Here's how the part is built. I have some questions about the finished solid (model axes, mm). A direction names the side the tool comes from. Coordinates: 2 decimals unless noted, no trailing zeros. Write each loop counter-clockwise with the first axis right and the second up, starting at its lowest first coordinate (ties: lowest second). Pieces come first, ordered by that corner, then holes.
(1) Thinking about a two-plate mould opening in X: for faces 1 (the flat face through (-2, -6, 1)), 2 (the cylindrical face through (-0.108, 5.812, 0.739)), 3 (the flat face through (5, -2, 1)), which applies, released by +X, released by -X, zero draft, split by the parting line, or undercut?
(2) Imagine slicing it at A-A, the plane x = -6.3. List the corners of the cut face in (y, z) for me, plus the area to 3 significant figures.
(3) Imagine slicing it at C-C, the plane z = -0.95. List the corners of the cut face in (x, y) for me, plus the area to 3 significant figures.
(4) Please list where these lines run through material, in increasing order: probe 1 along Y at (x, z) = (6.3, 0.5); probe 2 along Z at (x, y) = (9.25, 1.25); probe 3 along X at (y, z) = (0, -0.65).
(5) For pin 1 Ø2 at (x, z) = (-0.5, -1.5) entering from +Y; pin 2 Ø0.8 at (y, z) = (6, 1) entering from -X; pin 3 Ø3 at (x, y) = (0, -8) entering from -Z, each with a flat end and sliding along its axis, tell me the tip position at first contact or that it passes through.
(6) Imagine slicing it at D-D, the plane y = 0. State how many separate pieces and enclosed holes the cut face has, plus the area to 3 significant figures.
(7) Which directions (+Z, -Z, +X, -X, +Y, -Y) give clear straight access to the entire face, cutting with the end or side of a thin tool? Please do faces 4 (the flat face through (-6, -2, 1)), 5 (the flat face through (5, 2, 1)), 6 (the flat face through (2, -6, 1)), 7 (the flat face through (-6, 2, 1)).
```python
from build123d import *

# Parameters (mm, degrees)
COMPACT_HORN_CENTER_OD6P9_PROFILE_R        = 3.45
COMPACT_HORN_CENTER_OD6P9_DEPTH            = 1.5
HORIZONTAL_BLADES_ASSUMED_WIDTH4_PROFILE_W = 16.3
HORIZONTAL_BLADES_ASSUMED_WIDTH4_PROFILE_H = 4
HORIZONTAL_BLADES_ASSUMED_WIDTH4_DEPTH     = 1.5
VERTICAL_BLADES_ASSUMED_WIDTH4_PROFILE_W   = 4
VERTICAL_BLADES_ASSUMED_WIDTH4_PROFILE_H   = 16.3
VERTICAL_BLADES_ASSUMED_WIDTH4_DEPTH       = 1.5
ROUNDED_BLADE_TIPS_R                       = 2
ROUNDED_TIPS_SPAN20P3_DEPTH                = 1.5
HUB_PROJECTION2P5_TOTAL_HEIGHT4_START      = -2.5
HUB_PROJECTION2P5_TOTAL_HEIGHT4_PROFILE_R  = 3.45
HUB_PROJECTION2P5_TOTAL_HEIGHT4_DEPTH      = 2.5
PURCHASED_SPLINE_INTERNALS_OMITTED_START   = -50
PURCHASED_SPLINE_INTERNALS_OMITTED_PROFI_R = 2.55
PURCHASED_SPLINE_INTERNALS_OMITTED_DEPTH   = 65.570346598
UNMODIFIED_STOCK_PILOT_HOLES_START         = -50
UNMODIFIED_STOCK_PILOT_HOLES_PROFILE_R     = 0.5
UNMODIFIED_STOCK_PILOT_HOLES_DEPTH         = 65.570346598


with BuildPart() as part:
    # Compact_horn_center_OD6p9_profile → Compact_horn_center_OD6p9 (new body)
    with BuildSketch(Plane.XY):
        Circle(COMPACT_HORN_CENTER_OD6P9_PROFILE_R)
    extrude(amount=COMPACT_HORN_CENTER_OD6P9_DEPTH)

    # Horizontal_blades_assumed_width4_profile → Horizontal_blades_assumed_width4 (add)
    with BuildSketch(Plane.XY):
        Rectangle(HORIZONTAL_BLADES_ASSUMED_WIDTH4_PROFILE_W, HORIZONTAL_BLADES_ASSUMED_WIDTH4_PROFILE_H)
    extrude(amount=HORIZONTAL_BLADES_ASSUMED_WIDTH4_DEPTH)

    # Vertical_blades_assumed_width4_profile → Vertical_blades_assumed_width4 (add)
    with BuildSketch(Plane.XY):
        Rectangle(VERTICAL_BLADES_ASSUMED_WIDTH4_PROFILE_W, VERTICAL_BLADES_ASSUMED_WIDTH4_PROFILE_H)
    extrude(amount=VERTICAL_BLADES_ASSUMED_WIDTH4_DEPTH)

    # Rounded_blade_tips → Rounded_tips_span20p3 (add)
    with BuildSketch(Plane.XY):
        with Locations((8.15, 0)):
            Circle(ROUNDED_BLADE_TIPS_R)
        with Locations((-8.15, 0)):
            Circle(ROUNDED_BLADE_TIPS_R)
        with Locations((0, 8.15)):
            Circle(ROUNDED_BLADE_TIPS_R)
        with Locations((0, -8.15)):
            Circle(ROUNDED_BLADE_TIPS_R)
    extrude(amount=ROUNDED_TIPS_SPAN20P3_DEPTH)

    # Hub_projection2p5_total_height4_profile → Hub_projection2p5_total_height4 (add)
    with BuildSketch(Plane.XY.offset(HUB_PROJECTION2P5_TOTAL_HEIGHT4_START)):
        with Locations(Location((0, 0, 0), (0, 0, 215.43015836))):
            Circle(HUB_PROJECTION2P5_TOTAL_HEIGHT4_PROFILE_R)
    extrude(amount=HUB_PROJECTION2P5_TOTAL_HEIGHT4_DEPTH)

    # Purchased_spline_internals_omitted_profile → Purchased_spline_internals_omitted (cut, through all)
    with BuildSketch(Plane.XY.offset(PURCHASED_SPLINE_INTERNALS_OMITTED_START)):
        Circle(PURCHASED_SPLINE_INTERNALS_OMITTED_PROFI_R)
    extrude(amount=PURCHASED_SPLINE_INTERNALS_OMITTED_DEPTH, mode=Mode.SUBTRACT)

    # Unmodified_stock_pilot_holes_profile → Unmodified_stock_pilot_holes (cut, through all)
    with BuildSketch(Plane.XY.offset(UNMODIFIED_STOCK_PILOT_HOLES_START)):
        with Locations((-8.3, 0)):
            Circle(UNMODIFIED_STOCK_PILOT_HOLES_PROFILE_R)
        with Locations((-6.3, 0)):
            Circle(UNMODIFIED_STOCK_PILOT_HOLES_PROFILE_R)
        with Locations((-4.3, 0)):
            Circle(UNMODIFIED_STOCK_PILOT_HOLES_PROFILE_R)
        with Locations((4.3, 0)):
            Circle(UNMODIFIED_STOCK_PILOT_HOLES_PROFILE_R)
        with Locations((6.3, 0)):
            Circle(UNMODIFIED_STOCK_PILOT_HOLES_PROFILE_R)
        with Locations((8.3, 0)):
            Circle(UNMODIFIED_STOCK_PILOT_HOLES_PROFILE_R)
        with Locations((0, -8.3)):
            Circle(UNMODIFIED_STOCK_PILOT_HOLES_PROFILE_R)
        with Locations((0, -6.3)):
            Circle(UNMODIFIED_STOCK_PILOT_HOLES_PROFILE_R)
        with Locations((0, -4.3)):
            Circle(UNMODIFIED_STOCK_PILOT_HOLES_PROFILE_R)
        with Locations((0, 4.3)):
            Circle(UNMODIFIED_STOCK_PILOT_HOLES_PROFILE_R)
        with Locations((0, 6.3)):
            Circle(UNMODIFIED_STOCK_PILOT_HOLES_PROFILE_R)
        with Locations((0, 8.3)):
            Circle(UNMODIFIED_STOCK_PILOT_HOLES_PROFILE_R)
    extrude(amount=UNMODIFIED_STOCK_PILOT_HOLES_DEPTH, mode=Mode.SUBTRACT)


solid = part.part
```
Recorded:
1. face 1: released by -X
1. face 2: undercut
1. face 3: zero draft
2. outline: (-2, 0) - (-0.5, 0) - (-0.5, 1.5) - (-2, 1.5) - close; (0.5, 0) - (2, 0) - (2, 1.5) - (0.5, 1.5) - close
2. area: 4.50 mm2
3. outline: circle Ø6.9 at (0, 0); hole circle Ø5.1 at (0, 0)
3. area: 17.0 mm2
4. probe 1: y = -2 to -0.5, 0.5 to 2
4. probe 2: z = 0 to 1.5
4. probe 3: x = -3.45 to -2.55, 2.55 to 3.45
5. pin 1: stops at y = 3.45
5. pin 2: stops at x = -2
5. pin 3: stops at z = 0
6. separate pieces: 8
6. enclosed holes: 0
6. area: 18.3 mm2
7. face 4: +Z, -Z, -X, -Y
7. face 5: +Z, -Z, +X, +Y
7. face 6: +Z, -Z, +X, -Y
7. face 7: +Z, -Z, -X, +Y
